Verification items for the finished model (mm, model axes). Face numbers are marked on the shaded views. Give positions to 0.01 mm unless a question says otherwise; leave off trailing zeros. Write each loop counter-clockwise with the first axis right and the second up, starting at its lowest first coordinate (ties: lowest second). Pieces come first, ordered by that corner, then holes. Notation, with made-up numbers: (-23, -12.75) -> (-18, -12.75) arc R15 ccw to (-18, -7.75) -> close; hole circle Ø11 at (16.25, 47.5). An arc over 180 degrees is marked (long way). Use one line per item in the form item = value. Start each with the question number.
(1) Section check C-C, the plane z = -2.75. Record the cut outline in (x, y), plus the area to 3 significant figures.
(2) Release check for a two-part mould opening along Y. For the marked faces 1, 2 and 3 record: pulls with the +Y half, pulls with the -Y half, needs draft (parallel to the pull), parting line crosses it, or undercut.
(3) Scan lines: L1, parallel to Y at x = 0, z = -7; L2, parallel to Z at x = 2, y = 5.5; L3, parallel to X at y = 3.5, z = -12. Record each from-to range of solid material in increasing order.
(4) Section check D-D, the plane z = -9.5. Record the cut outline in (x, y), plus the area to 3 significant figures.
(5) Depth check by flat-ended pin: pin 1 Ø1.5 at (y, z) = (-2, -3.5) entering from +X; pin 2 Ø5.5 at (x, y) = (0, 0) entering from +Z; pin 3 Ø5 at (x, y) = (-5.5, 5.5) entering from -Z; pin 4 Ø8 at (y, z) = (1.5, -12.5) entering from +X. Enter the tip coordinate at first touch or a pass-through.
from build123d import *

# Parameters (mm, degrees)
F0_R     = 5.5
F0_R_2   = 4.5
F1_DEPTH = 15
F0_R_3   = 7.5
F2_DEPTH = 5
F3_R     = 0.99999


# Not quite as in the source:
# - a fillet or chamfer is up to 0.001 mm smaller than in the source, because OpenCascade refuses the exact size


with BuildPart() as f1:
    # F0 (on Top) → F1 (new body)
    with BuildSketch(Plane.XY):
        Circle(F0_R)
        Circle(F0_R_2, mode=Mode.SUBTRACT)
    extrude(amount=-F1_DEPTH)

    # F0 (on Top) → F2 (join)
    with BuildSketch(Plane.XY):
        Circle(F0_R_3)
        Circle(F0_R, mode=Mode.SUBTRACT)
    extrude(amount=-F2_DEPTH)

    # F3 (radius 1 in the source; OpenCascade refuses exactly that, so slightly less here)
    f3_edges = [f1.edges().sort_by_distance(p)[0] for p in [
        (-7.5, 0, 0),
        (-5.5, 0, -15),
    ]]
    fillet(f3_edges, radius=F3_R)


solid = f1.part
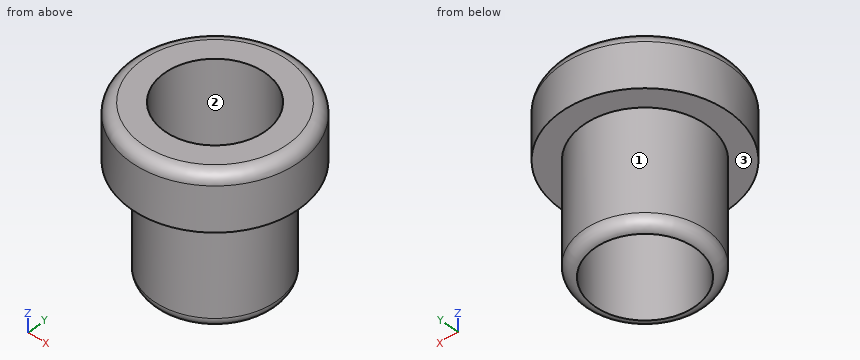
Completed:
q1.outline = circle Ø15 at (0, 0); hole circle Ø9 at (0, 0)
q1.area = 113 mm²
q2.face_1 = parting line crosses it
q2.face_2 = undercut
q2.face_3 = needs draft
q3.L1 = -5.5 to -4.5, 4.5 to 5.5
q3.L2 = -5 to 0
q3.L3 = -4.24 to -2.83, 2.83 to 4.24
q4.outline = circle Ø11 at (0, 0); hole circle Ø9 at (0, 0)
q4.area = 31.4 mm²
q5.pin_1 = 7.4
q5.pin_2 = through
q5.pin_3 = -14.63
q5.pin_4 = 5.5
